Build history of the part. All positions in model axes, mm. A direction names the side the tool comes from. Coordinates: 2 decimals unless noted, no trailing zeros. Order: outer loops, then holes, each group sorted by start corner. A loop starts at its lowest first (then second) coordinate and runs counter-clockwise, first axis right, second up. Notation, with made-up numbers: (74, -15.75) - (124, -15.75) arc R19 ccw to (124, -3.75) - close; hole circle Ø5 at (-24, 89). An arc over 180 degrees is marked (long way). Return JSON: item names as keys, results as strings.
from build123d import *

# Parameters (mm, degrees)
EXTRUSION1_DEPTH                = 70
ESQUISSE2_R                     = 1.5
EXTRUSION2_DEPTH                = 98.549987186
R_P_TITION_LIN_AIRE1_COUNT      = 2
R_P_TITION_LIN_AIRE1_PITCH      = 50
R_P_TITION_LIN_AIRE1_COUNT_DIR2 = 2
R_P_TITION_LIN_AIRE1_PITCH_DIR2 = 25
ESQUISSE3_R                     = 2
ENL_V_MAT_EXTRU_1_DEPTH         = 10


with BuildPart() as part:
    # Esquisse1 → Extrusion1 (new body)
    with BuildSketch(Plane.XY):
        Polygon((0, 0), (4, 0), (50, 0), (50, 4), (4, 4), (4, 50), (0, 50), align=None)
    extrude(amount=EXTRUSION1_DEPTH)

    # Esquisse2 → Extrusion2 (cut, through all)
    with BuildSketch(Plane(origin=(0, 4, 0), x_dir=(1, 0, 0), z_dir=(0, 1, 0))):
        with Locations(Location((40, -60, 0), (0, 0, 270))):
            Circle(ESQUISSE2_R)
    extrusion2 = extrude(amount=-EXTRUSION2_DEPTH, mode=Mode.SUBTRACT)

    # Répétition linéaire1: Extrusion2 2 × 2
    with Locations(*[(-j * R_P_TITION_LIN_AIRE1_PITCH_DIR2, 0, -i * R_P_TITION_LIN_AIRE1_PITCH) for i in range(R_P_TITION_LIN_AIRE1_COUNT) for j in range(R_P_TITION_LIN_AIRE1_COUNT_DIR2) if (i, j) != (0, 0)]):
        add(extrusion2, mode=Mode.SUBTRACT)

    # Esquisse3 → Enlèv. mat.-Extru.1 (cut)
    with BuildSketch(Plane.ZY):
        with Locations((24.65, 40)):
            Circle(ESQUISSE3_R)
    extrude(amount=-ENL_V_MAT_EXTRU_1_DEPTH, mode=Mode.SUBTRACT)


solid = part.part
1. Cut at C-C on x = 40. Give the cut face in (y, z), plus the area to 3 significant figures.
Check values:
{"outline": "(0, 0) - (4, 0) - (4, 8.5) - (0, 8.5) - close; (0, 11.5) - (4, 11.5) - (4, 58.5) - (0, 58.5) - close; (0, 61.5) - (4, 61.5) - (4, 70) - (0, 70) - close", "area": "256 mm²"}
2. Cut at A-A on y = 40. Give the cut face in (x, z).
Check values:
{"outline": "(0, 0) - (4, 0) - (4, 22.65) - (0, 22.65) - close; (0, 26.65) - (4, 26.65) - (4, 70) - (0, 70) - close"}
3. Cut at D-D on z = 24.65. Give the cut face in (x, y).
Check values:
{"outline": "(0, 0) - (50, 0) - (50, 4) - (4, 4) - (4, 38) - (0, 38) - close; (0, 42) - (4, 42) - (4, 50) - (0, 50) - close"}
4. Tool access for faces 1 (the flat face through (4, 27, 35)), 2 (the flat face through (25, 0, 35)): list every direction of +Z, -Z, +X, -X, +Y, -Y with a clear straight run to the whole face (end or side of a thin tool).
Check values:
{"face 1": "+Z, -Z, +X, +Y", "face 2": "+Z, -Z, +X, -X, -Y"}
5. Cut at B-B on z = 10. Give the cut face in (x, y), plus the area to 3 significant figures.
Check values:
{"outline": "(0, 0) - (13.5, 0) - (13.5, 4) - (4, 4) - (4, 50) - (0, 50) - close; (16.5, 0) - (38.5, 0) - (38.5, 4) - (16.5, 4) - close; (41.5, 0) - (50, 0) - (50, 4) - (41.5, 4) - close", "area": "360 mm²"}
6. Mould opens along Z. For faces 3 (the cylindrical face through (38.536, 2.028, 9.675)), 4 (the cylindrical face through (1.972, 38.226, 25.573)), 5 (the flat face through (0, 25, 35)), 6 (the flat face through (3, 14, 70)) say: pulls with the +Z half, pulls with the -Z half, needs draft (parallel to the pull), parting line crosses it, or undercut.
Check values:
{"face 3": "undercut", "face 4": "undercut", "face 5": "needs draft", "face 6": "pulls with the +Z half"}
7. Probe L1, parallel to X at y = 1, z = 10; L2, parallel to X at y = 47, z = 20; L3, parallel to Y at x = 2, z = 24. List the from-to ranges inside material, lowest first.
Check values:
{"L1": "0 to 13.5, 16.5 to 38.5, 41.5 to 50", "L2": "0 to 4", "L3": "0 to 38.11, 41.89 to 50"}
8. Drop flat-ended pins along their axis: pin 1 (12 mm diameter, centred on y = 25.5, z = 31.5, fed in from -X); pin 2 (3 mm diameter, centred on x = 32.5, z = 56, fed in from +Y); pin 3 (1.5 mm diameter, centred on y = 17.5, z = 42, fed in from +X). Give the stop position or say it passes through.
Check values:
{"pin 1": "x = 0", "pin 2": "y = 4", "pin 3": "x = 4"}
